from build123d import *

# Parameters (mm, degrees)
SKETCH_1_W          = 10
SKETCH_1_H          = 10
SKETCH_1_W_2        = 8
SKETCH_1_H_2        = 8
EXTRUDE_1_DEPTH     = 172
SKETCH_2_R          = 1.6
CUT_EXTRUDE_1_DEPTH = 173.362989067


with BuildPart() as part:
    # ｽｹｯﾁ1 → 押し出し-薄板1 (new body)
    with BuildSketch(Plane(origin=(0, 0, 0), x_dir=(0, 0, -1), z_dir=(1, 0, 0))):
        Rectangle(SKETCH_1_W, SKETCH_1_H)
        Rectangle(SKETCH_1_W_2, SKETCH_1_H_2, mode=Mode.SUBTRACT)
    extrude(amount=EXTRUDE_1_DEPTH)

    # ｽｹｯﾁ2 → ｶｯﾄ - 押し出し1 (cut, through all)
    with BuildSketch(Plane.XY.offset(5)):
        with Locations((15, 0)):
            Circle(SKETCH_2_R)
        with Locations((5, 0)):
            Circle(SKETCH_2_R)
        with Locations(Location((167, 0, 0), (0, 0, 90))):
            Circle(SKETCH_2_R)
        with Locations(Location((157, 0, 0), (0, 0, 90))):
            Circle(SKETCH_2_R)
    extrude(amount=-CUT_EXTRUDE_1_DEPTH, mode=Mode.SUBTRACT)


solid = part.part
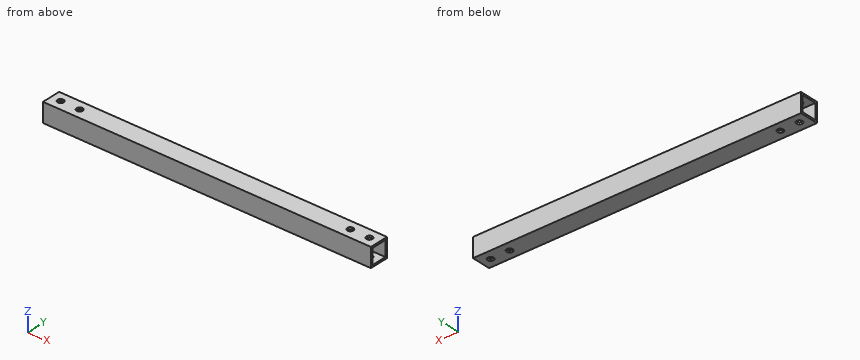
Could you check a few things on this model? Use its own coordinates, in mm. Give positions to 0.01 mm unless a question says otherwise; leave off trailing zeros. Loops run counter-clockwise (first coordinate to the right, second up) from the corner with the lowest first, then second, coordinate; pieces in that order, holes last. Notation, with made-up numbers: (23, 15.25) -> (76, 15.25) arc R14 cw to (76, 27.25) -> close; hole circle Ø2 at (39, -28.75). An arc over 180 degrees is marked (long way). Return JSON: item names as keys, results as strings.
Item 1: If we section it at A-A on x = 157: List the corners of the cut face in (y, z) for me, plus the area to 3 significant figures.
Geometry results:
{"outline": "(-5, -5) -> (-1.6, -5) -> (-1.6, -4) -> (-4, -4) -> (-4, 4) -> (-1.6, 4) -> (-1.6, 5) -> (-5, 5) -> close; (1.6, -5) -> (5, -5) -> (5, 5) -> (1.6, 5) -> (1.6, 4) -> (4, 4) -> (4, -4) -> (1.6, -4) -> close", "area": "29.6 mm²"}
Item 2: If we section it at B-B on z = -0.5: List the corners of the cut face in (x, y) for me.
Geometry results:
{"outline": "(0, -5) -> (172, -5) -> (172, -4) -> (0, -4) -> close; (0, 4) -> (172, 4) -> (172, 5) -> (0, 5) -> close"}
Item 3: I need wall thicknesses on L1, parallel to Z at x = 41, y = -0.25; L2, parallel to Y at x = 167, z = -4.8. Which ranges of each line are inside material? Lowest first, please. Write a range as from..to.
Geometry results:
{"L1": "z = -5..-4, 4..5", "L2": "y = -5..-1.6, 1.6..5"}
Item 4: If we section it at C-C on x = 70: List the corners of the cut face in (y, z) for me.
Geometry results:
{"outline": "(-5, -5) -> (5, -5) -> (5, 5) -> (-5, 5) -> close; hole (-4, -4) -> (4, -4) -> (4, 4) -> (-4, 4) -> close"}
Item 5: If we section it at D-D on y = 0: Count the separate pieces of the cut face and the enclosed holes in it, plus the area to 3 significant figures.
Geometry results:
{"separate pieces": "10", "enclosed holes": "0", "area": "318 mm²"}
